```python
from build123d import *

# Parameters (mm, degrees)
SKETCH1_W                           = 38.1
SKETCH1_H                           = 7.9375
BOSS_EXTRUDE1_DEPTH                 = 39.624
SKETCH2_W                           = 19.05
SKETCH2_H                           = 2.54
CUT_EXTRUDE1_DEPTH                  = 45.144250504
F_1_8_0_125_CLEARANCE_DOWEL_HOLE1_D = 3.175
SKETCH6_W                           = 4.7625
SKETCH6_H                           = 7.9375
CUT_EXTRUDE2_DEPTH                  = 3.175


with BuildPart() as part:
    # Sketch1 → Boss-Extrude1 (new body)
    with BuildSketch(Plane.XY):
        Rectangle(SKETCH1_W, SKETCH1_H)
    extrude(amount=BOSS_EXTRUDE1_DEPTH)

    # Sketch2 → Cut-Extrude1 (cut, through all)
    with BuildSketch(Plane.XY.offset(39.624)):
        with Locations((0, 2.69875)):
            Rectangle(SKETCH2_W, SKETCH2_H)
    extrude(amount=-CUT_EXTRUDE1_DEPTH, mode=Mode.SUBTRACT)

    # 1/8 (0.125) Clearance Dowel Hole1 (through all)
    with Locations(Plane(origin=(0, 0, 0), x_dir=(-1, 0, 0), z_dir=(0, 0, -1))):
        with Locations((-16.66875, 0.79375), (16.66875, 0.79375)):
            Hole(F_1_8_0_125_CLEARANCE_DOWEL_HOLE1_D / 2)

    # Sketch6 → Cut-Extrude2 (cut)
    with BuildSketch(Plane.XY.offset(39.624)):
        with Locations((-16.66875, 0)):
            Rectangle(SKETCH6_W, SKETCH6_H)
        with Locations((16.66875, 0)):
            Rectangle(SKETCH6_W, SKETCH6_H)
    extrude(amount=-CUT_EXTRUDE2_DEPTH, mode=Mode.SUBTRACT)


solid = part.part
```
Here's how the part is built. I have some questions about the finished solid (model axes, mm). A direction names the side the tool comes from. Round coordinates to 2 decimals unless told otherwise and drop trailing zeros. Order: outer loops, then holes, each group sorted by start corner. A loop starts at its lowest first (then second) coordinate and runs counter-clockwise, first axis right, second up. Notation, with made-up numbers: (58, 32.25) -> (113, 32.25) arc R26 ccw to (113, 49.25) -> close; hole circle Ø8 at (77.5, -19). An arc over 180 degrees is marked (long way). Use a Markdown table: item, result. Add a question column.
(1) Suppose I cut it at D-D, the plane x = 2. Please give me the cut outline in (y, z), and give its area (3 significant figures).
(2) For faces 4 (the face through (-17, -1, 36.449)), 5 (the face through (14.288, 0, 38)), 6 (the face through (0, 1.429, 20)), which set-ups out of +Z, -Z, +X, -X, +Y, -Y let a thin tool reach every point of the face, with its end or its side?
(3) Suppose I cut it at B-B, the plane y = -1.75. Please give me the cut outline in (x, z), and give its area (3 significant figures).
(4) Suppose I cut it at C-C, the plane z = 29. Count the separate pieces of the cut face and the enclosed holes in it, and give its area (3 significant figures).
(5) I need wall thicknesses on line 1 along X through (y, z) = (0.75, 31.5); line 2 along X through (y, z) = (3.5, 5.5) (3 decimals); line 3 along X through (y, z) = (1, 31). Which ranges of each line are inside material? Lowest first, please.
(6) Suppose I cut it at A-A, the plane x = -16. Please give me the cut outline in (y, z), and give its area (3 significant figures).
(7) If we mould it in two halves opening along X, with no side actions, what happens to faces 1 (the face through (0, -3.969, 20)), 2 (the face through (19.05, 0, 18)), 3 (the face through (17.522, 2.132, 18.48))? For each: released by +X, released by -X, zero draft, split by the parting line, or undercut.
(8) For pin 1 Ø1.6 at (y, z) = (0.5, 39) entering from -X; pin 2 Ø1.9 at (x, y) = (-16.67, 0.79) entering from +Z; pin 3 Ø2.5 at (y, z) = (0.5, 38.5) entering from +X; pin 4 Ø2.5 at (x, y) = (-17, 0) entering from +Z, each with a flat end and sliding along its axis, tell me the tip position at first contact or that it passes through.
Verdict:
| question | item | result |
|---|---|---|
| 1 | outline | (-3.97, 0) -> (1.43, 0) -> (1.43, 39.62) -> (-3.97, 39.62) -> close |
| 1 | area | 214 mm2 |
| 2 | face 4 | +Z, -X, +Y, -Y |
| 2 | face 5 | +Z, +X, +Y, -Y |
| 2 | face 6 | +Z, -Z, +Y |
| 3 | outline | (-19.05, 0) -> (19.05, 0) -> (19.05, 36.45) -> (14.29, 36.45) -> (14.29, 39.62) -> (-14.29, 39.62) -> (-14.29, 36.45) -> (-19.05, 36.45) -> close |
| 3 | area | 1,480 mm2 |
| 4 | separate pieces | 1 |
| 4 | enclosed holes | 2 |
| 4 | area | 238 mm2 |
| 5 | line 1 | -19.05 to -18.26, -15.08 to 15.08, 18.26 to 19.05 |
| 5 | line 2 | -19.05 to -9.525, 9.525 to 19.05 |
| 5 | line 3 | -19.05 to -18.24, -15.09 to 15.09, 18.24 to 19.05 |
| 6 | outline | (-3.97, 0) -> (-0.65, 0) -> (-0.65, 36.45) -> (-3.97, 36.45) -> close; (2.23, 0) -> (3.97, 0) -> (3.97, 36.45) -> (2.23, 36.45) -> close |
| 6 | area | 184 mm2 |
| 7 | face 1 | zero draft |
| 7 | face 2 | released by +X |
| 7 | face 3 | undercut |
| 8 | pin 1 | x = -14.29 |
| 8 | pin 2 | through |
| 8 | pin 3 | x = 14.29 |
| 8 | pin 4 | z = 36.45 |
